Here's how the part is built. I have some questions about the finished solid (model axes, mm). A direction names the side the tool comes from. Give positions to 0.01 mm unless a question says otherwise; leave off trailing zeros. Loops run counter-clockwise (first coordinate to the right, second up) from the corner with the lowest first, then second, coordinate; pieces in that order, holes last. Notation, with made-up numbers: M -1.75,-37 L 6.25,-37 A11 ccw 6.25,-18 Z; hole C -10,-32 d8. An arc over 180 degrees is marked long. Write item = value, one per line. Start each with the question number.
```python
from build123d import *

# Parameters (mm, degrees)
SKETCH1_W           = 30
SKETCH1_H           = 30
BOSS_EXTRUDE1_DEPTH = 171
SKETCH2_R           = 10
CUT_EXTRUDE1_DEPTH  = 10
SKETCH3_W           = 30
SKETCH3_H           = 30
BOSS_EXTRUDE2_DEPTH = 37.6839
SKETCH5_W           = 30
SKETCH5_H           = 30
BOSS_EXTRUDE3_DEPTH = 10


with BuildPart() as part:
    # Sketch1 → Boss-Extrude1 (new body)
    with BuildSketch(Plane(origin=(0, 0, 0), x_dir=(1, 0, 0), z_dir=(0, 1, 0))):
        Rectangle(SKETCH1_W, SKETCH1_H)
    extrude(amount=BOSS_EXTRUDE1_DEPTH)

    # Sketch2 → Cut-Extrude1 (cut)
    with BuildSketch(Plane.XZ):
        Circle(SKETCH2_R)
    extrude(amount=-CUT_EXTRUDE1_DEPTH, mode=Mode.SUBTRACT)

    # Sketch3 → Boss-Extrude2 (add)
    with BuildSketch(Plane.XY.offset(15)):
        with Locations((0, 156)):
            Rectangle(SKETCH3_W, SKETCH3_H)
    extrude(amount=BOSS_EXTRUDE2_DEPTH)

    # Sketch5 → Boss-Extrude3 (add)
    with BuildSketch(Plane(origin=(0, 171, 0), x_dir=(1, 0, 0), z_dir=(0, 1, 0))):
        with Locations((0, -37.6839)):
            Rectangle(SKETCH5_W, SKETCH5_H)
    extrude(amount=BOSS_EXTRUDE3_DEPTH)


solid = part.part
```
Q1. Will these pins go through, and if not, where does the flat tip stop? pin 1 (16 mm diameter, centred on x = 0, z = 0, fed in from -Y); pin 2 (15 mm diameter, centred on x = 0.5, z = 36.5, fed in from -Y); pin 3 (4 mm diameter, centred on x = 8.5, y = 112.5, fed in from +Z).
Q2. If we section it at D-D, the plane z = 20.5: List the corners of the cut face in (x, y) for me, then the cut area to 3 significant figures.
Q3. If we section it at A-A, the plane z = 0: List the corners of the cut face in (x, y) for me, then the cut area to 3 significant figures.
Q4. On a 3-axis mill with a long thin cutter (end or side, diameter ignored), from which of +Z, -Z, +X, -X, +Y, -Y can I reach the whole of each face in a straight line? I mean faces 1 (the cylindrical face through (-2.17, 4.93, -9.76)), 2 (the flat face through (-0.2, 0, -10.2)), 3 (the flat face through (0, 141, 34)). Say none if no direction works.
Q5. If we section it at B-B, the plane x = 0: List the corners of the cut face in (y, z) for me.
Q6. We'd pull the mould along Z, two halves only. Please class faces 4 (the flat face through (0, 161, 52.684)), 5 (the flat face through (0, 176, 22.684)), 6 (the flat face through (0, 171, 4)), 7 (the flat face through (0, 10, 0)): pulls with the +Z half, pulls with the -Z half, needs draft (parallel to the pull), parting line crosses it, or undercut.
Q7. If I drill on line 1 along Z through (x, y) = (0, 2.5); line 2 along Y through (x, z) = (2.25, 35); line 3 along Z through (x, y) = (8.25, 115), over which ranges is the centre line in solid material (lowest first)?
Q8. If we section it at C-C, the plane y = 93.5: List the corners of the cut face in (x, z) for me, then the cut area to 3 significant figures.
Resolved:
q1.pin_1 = 10
q1.pin_2 = 141
q1.pin_3 = 15
q2.outline = M -15,141 L 15,141 L 15,171 L -15,171 Z
q2.area = 900 mm²
q3.outline = M -15,0 L -10,0 L -10,10 L 10,10 L 10,0 L 15,0 L 15,171 L -15,171 Z
q3.area = 4,930 mm²
q4.face_1 = -Y
q4.face_2 = +Z, -Z, +X, -X, -Y
q4.face_3 = +Z, +X, -X, -Y
q5.outline = M 0,-15 L 171,-15 L 171,22.68 L 181,22.68 L 181,52.68 L 141,52.68 L 141,15 L 0,15 L 0,10 L 10,10 L 10,-10 L 0,-10 Z
q6.face_4 = pulls with the +Z half
q6.face_5 = pulls with the -Z half
q6.face_6 = needs draft
q6.face_7 = undercut
q7.line_1 = -15 to -10, 10 to 15
q7.line_2 = 141 to 181
q7.line_3 = -15 to 15
q8.outline = M -15,-15 L 15,-15 L 15,15 L -15,15 Z
q8.area = 900 mm²
